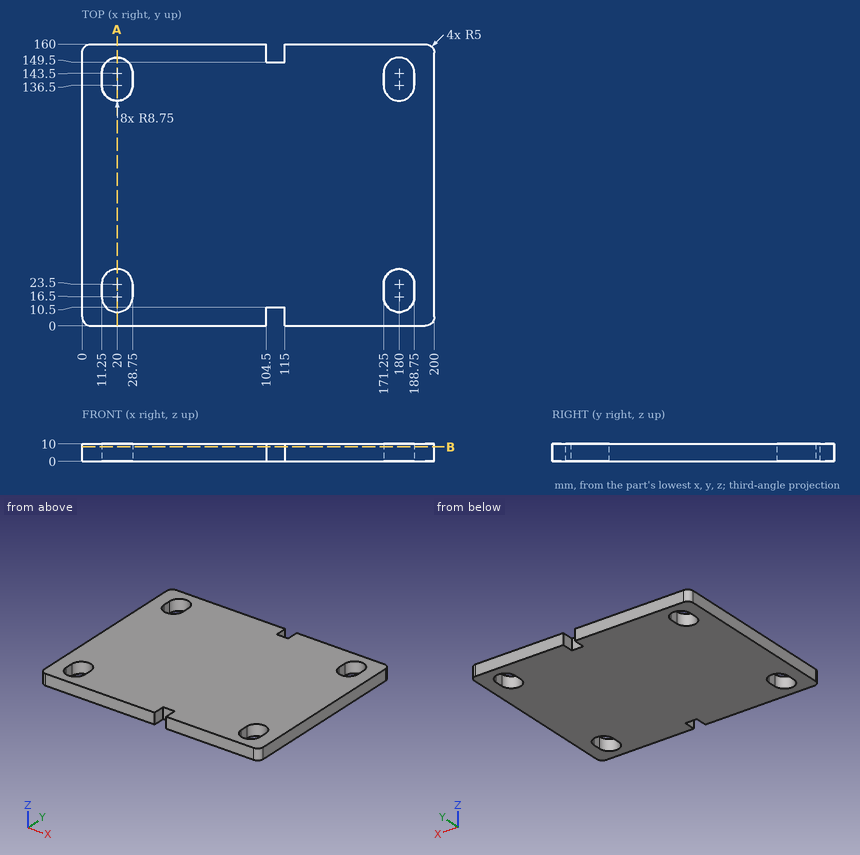
Here's the drawing with two shaded views (mm, measured from the low corner). I have some questions. Give positions to 0.01 mm unless a question says otherwise; leave off trailing zeros. Write each loop counter-clockwise with the first axis right and the second up, starting at its lowest first coordinate (ties: lowest second). Pieces come first, ordered by that corner, then holes. Notation, with made-up numbers: (-18, 80.5) - (-9, 80.5) arc R20 ccw to (-9, 91.5) - close; hole circle Ø5 at (46.25, -31.75). An arc over 180 degrees is marked (long way). Write item = value, one per line. Start each with the question number.
1. Please list where these lines run through material, in increasing order: line 1 (X direction, y = 24, z = 8); line 2 (Y direction, x = 15, z = 8); line 3 (Y direction, x = 187.5, z = 9.5).
2. Imagine slicing it at A-A (x = 20). Please give me the cut outline in (y, z).
3. For pin 1 (2 mm diameter, centred on y = 140.5, z = 6, fed in from -X), with a flat end and sliding along its axis, tell me the tip position at first contact or that it passes through.
4. Imagine slicing it at B-B (z = 8.25). Count the separate pieces of the cut face and the enclosed holes in it, and give its area (3 significant figures).
Worked answers:
q1.line_1 = 0 to 11.26, 28.74 to 171.26, 188.74 to 200
q1.line_2 = 0 to 9.32, 30.68 to 129.32, 150.68 to 160
q1.line_3 = 0 to 11.99, 28.01 to 131.99, 148.01 to 160
q2.outline = (0, 0) - (7.75, 0) - (7.75, 10) - (0, 10) - close; (32.25, 0) - (127.75, 0) - (127.75, 10) - (32.25, 10) - close; (152.25, 0) - (160, 0) - (160, 10) - (152.25, 10) - close
q3.pin_1 = 0
q4.separate_pieces = 1
q4.enclosed_holes = 4
q4.area = 30,300 mm2
